```python
from build123d import *

# Parameters (mm, degrees)
F0_R      = 15
F1_DEPTH  = 22.5
F2_DEPTH  = 8.5
F5_W      = 10
F5_H      = 50
F6_DEPTH  = 31
F8_R      = 15
F9_DEPTH  = 16
F10_DEPTH = 14
F12_DEPTH = 4


# Not quite as in the source:
# - a pattern or mirror of a feature is missing from the dataset's text; its kind, count and spacing are read off the source's solid


with BuildPart() as f1:
    # F0 (on Front) → F1 (new body, symmetric)
    with BuildSketch(Plane.XZ):
        with BuildLine():
            ThreePointArc((0, -25), (17.6776695297, -17.6776695297), (25, 0))
            ThreePointArc((25, 0), (17.6776695297, 17.6776695297), (0, 25))
            ThreePointArc((0, 25), (-25, 0), (0, -25))
        make_face()
        Circle(F0_R, mode=Mode.SUBTRACT)
    extrude(amount=F1_DEPTH, both=True)

    # F0 (on Front) → F2 (join, symmetric)
    with BuildSketch(Plane.XZ):
        with BuildLine():
            ThreePointArc((0, 25), (17.6776695297, 17.6776695297), (25, 0))
            ThreePointArc((25, 0), (17.6776695297, -17.6776695297), (0, -25))
            Line((0, -25), (70, -25))
            Line((70, -25), (70, 25))
            Line((70, 25), (0, 25))
        make_face()
    extrude(amount=F2_DEPTH, both=True)

    # F5 (on Front) → F6 (join, symmetric)
    with BuildSketch(Plane.XZ):
        with Locations((75, 0)):
            Rectangle(F5_W, F5_H)
    extrude(amount=F6_DEPTH, both=True)

    # F8 (on face) → F9 (join)
    with BuildSketch(Plane.XZ.offset(31)):
        with BuildLine():
            Line((93.4168760482, 25), (80, 25))
            Line((80, 25), (80, 0))
            ThreePointArc((80, 0), (83.5661796315, 14.1863716546), (93.4168760482, 25))
        make_face()
        with BuildLine():
            ThreePointArc((93.4168760482, 25), (83.5661796315, 14.1863716546), (80, 0))
            ThreePointArc((80, 0), (83.5661796315, -14.1863716546), (93.4168760482, -25))
            ThreePointArc((93.4168760482, -25), (124.1863716546, -26.4338203685), (140, 0))
            ThreePointArc((140, 0), (124.1863716546, 26.4338203685), (93.4168760482, 25))
        make_face()
        with Locations((110, 0)):
            Circle(F8_R, mode=Mode.SUBTRACT)
        with BuildLine():
            ThreePointArc((93.4168760482, -25), (83.5661796315, -14.1863716546), (80, 0))
            Line((80, 0), (80, -25))
            Line((80, -25), (93.4168760482, -25))
        make_face()
    f9 = extrude(amount=-F9_DEPTH)

    # F9_copies: F9 across plane
    add(f9.mirror(Plane.ZX))

    # F8 (on face) → F10 (join)
    with BuildSketch(Plane.XZ.offset(31)):
        with BuildLine():
            Line((93.4168760482, 25), (80, 25))
            Line((80, 25), (80, 0))
            ThreePointArc((80, 0), (83.5661796315, 14.1863716546), (93.4168760482, 25))
        make_face()
        with BuildLine():
            ThreePointArc((93.4168760482, -25), (83.5661796315, -14.1863716546), (80, 0))
            Line((80, 0), (80, -25))
            Line((80, -25), (93.4168760482, -25))
        make_face()
        with BuildLine():
            ThreePointArc((93.4168760482, 25), (83.5661796315, 14.1863716546), (80, 0))
            ThreePointArc((80, 0), (83.5661796315, -14.1863716546), (93.4168760482, -25))
            ThreePointArc((93.4168760482, -25), (124.1863716546, -26.4338203685), (140, 0))
            ThreePointArc((140, 0), (124.1863716546, 26.4338203685), (93.4168760482, 25))
        make_face()
        with Locations((110, 0)):
            Circle(F8_R, mode=Mode.SUBTRACT)
    extrude(amount=-F10_DEPTH)

    # F8 (on face) → F12 (join)
    with BuildSketch(Plane.XZ.offset(31)):
        with BuildLine():
            ThreePointArc((93.4168760482, 25), (83.5661796315, 14.1863716546), (80, 0))
            ThreePointArc((80, 0), (83.5661796315, -14.1863716546), (93.4168760482, -25))
            ThreePointArc((93.4168760482, -25), (124.1863716546, -26.4338203685), (140, 0))
            ThreePointArc((140, 0), (124.1863716546, 26.4338203685), (93.4168760482, 25))
        make_face()
        with Locations((110, 0)):
            Circle(F8_R, mode=Mode.SUBTRACT)
    f12 = extrude(amount=F12_DEPTH)

    # F12_copies: F12 across plane
    add(f12.mirror(Plane.ZX))


solid = f1.part
```
Can you work these out from the model? Positions are in its coordinate system, mm. A direction names the side the tool comes from. Coordinates: 2 decimals unless noted, no trailing zeros. Loops run counter-clockwise (first coordinate to the right, second up) from the corner with the lowest first, then second, coordinate; pieces in that order, holes last.
1) Which directions (+Z, -Z, +X, -X, +Y, -Y) give clear straight access to the entire face, cutting with the end or side of a thin tool? Please do faces 4 (the flat face through (11, 22.5, -11)), 5 (the flat face through (11, -22.5, -11)), 6 (the flat face through (70, -20, 0)).
2) Thinking about a two-plate mould opening in X: for faces 1 (the flat face through (116, 35, 14)), 2 (the flat face through (80, 0, 0)), 3 (the flat face through (70, 20, 0)), which applies, pulls with the +X half, pulls with the -X half, needs draft (parallel to the pull), parting line crosses it, or undercut?
3) Imagine slicing it at C-C on z = -3.5. State how many separate pieces and enclosed holes the cut face has, plus the area to 3 significant figures.
4) Imagine slicing it at A-A on x = 110. List the corners of the cut face in (y, z) for me.
5) For pin 1 (1 mm diameter, centred on x = 0.5, y = 24, fed in from -Z); pin 2 (4 mm diameter, centred on x = 51, z = -15, fed in from +Y); pin 3 (12 mm diameter, centred on x = 76.5, y = 28, fed in from +Z); pin 4 (2 mm diameter, centred on y = -13, z = 5, fed in from +X), each with a flat end and sliding along its axis, tell me the tip position at first contact or that it passes through.
6) Imagine slicing it at D-D on x = 8.5. List the corners of the cut face in (y, z) for me, plus the area to 3 significant figures.
7) Imagine slicing it at B-B on y = 19. List the corners of the cut face in (x, z) for me.
8) I need wall thicknesses on probe 1 along Y at (x, z) = (113, -26); probe 2 along Z at (x, y) = (110, -27.5); probe 3 along X at (y, z) = (-11, 1.5). Which ranges of each line are inside material? Lowest first, please.
Completed:
1. face 4: +Z, -Z, -X, +Y
1. face 5: +Z, -Z, -X, -Y
1. face 6: +Z, -Z, -Y
2. face 1: needs draft
2. face 2: pulls with the +X half
2. face 3: undercut
3. separate pieces: 4
3. enclosed holes: 0
3. area: 3,530 mm2
4. outline: (-35, -30) - (-15, -30) - (-15, -15) - (-35, -15) - close; (-35, 15) - (-15, 15) - (-15, 30) - (-35, 30) - close; (15, -30) - (35, -30) - (35, -15) - (15, -15) - close; (15, 15) - (35, 15) - (35, 30) - (15, 30) - close
5. pin 1: passes through
5. pin 2: stops at y = 8.5
5. pin 3: stops at z = 25
5. pin 4: stops at x = 80
6. outline: (-22.5, -23.51) - (-8.5, -23.51) - (-8.5, -25) - (8.5, -25) - (8.5, -23.51) - (22.5, -23.51) - (22.5, -12.36) - (-22.5, -12.36) - close; (-22.5, 12.36) - (22.5, 12.36) - (22.5, 23.51) - (8.5, 23.51) - (8.5, 25) - (-8.5, 25) - (-8.5, 23.51) - (-22.5, 23.51) - close
6. area: 1,050 mm2
7. outline: circle Ø50 at (0, 0); (70, -25) - (93.42, -25) arc R30 ccw (long way) to (93.42, 25) - (70, 25) - close; hole circle Ø30 at (0, 0); hole circle Ø30 at (110, 0)
8. probe 1: y = -35 to -15, 15 to 35
8. probe 2: z = -30 to -15, 15 to 30
8. probe 3: x = -24.95 to -14.92, 14.92 to 24.95, 70 to 80
